```python
from build123d import *

# Parameters (mm, degrees)
BOSS_EXTRUDE1_DEPTH     = 2.54
SKETCH2_W               = 100.584
SKETCH2_H               = 101.6
BOSS_EXTRUDE2_DEPTH     = 152.4
SKETCH4_W               = 97.79508
SKETCH4_H               = 98.81108
CUT_EXTRUDE1_DEPTH      = 190.5
SKETCH6_R               = 3.175
CUT_EXTRUDE2_DEPTH      = 203.856506729
CUT_EXTRUDE4_DEPTH      = 82.182271537
CUT_EXTRUDE4_DEPTH_BACK = 183.782271537


with BuildPart() as part:
    # Sketch1 → Boss-Extrude1 (new body)
    with BuildSketch(Plane(origin=(0, 0, 0), x_dir=(1, 0, 0), z_dir=(0, 1, 0))):
        Polygon((76.035493271, -131.982271537), (152.235493271, 0), (76.035493271, 131.982271537), (-76.364506729, 131.982271537), (-152.564506729, 0), (-76.364506729, -131.982271537), align=None)
    extrude(amount=BOSS_EXTRUDE1_DEPTH)

    # Sketch2 → Boss-Extrude2 (add)
    with BuildSketch(Plane(origin=(0, 2.54, 0), x_dir=(1, 0, 0), z_dir=(0, 1, 0))):
        Rectangle(SKETCH2_W, SKETCH2_H)
    extrude(amount=BOSS_EXTRUDE2_DEPTH)

    # Sketch4 → Cut-Extrude1 (cut)
    with BuildSketch(Plane(origin=(0, 154.94, 0), x_dir=(1, 0, 0), z_dir=(0, 1, 0))):
        Rectangle(SKETCH4_W, SKETCH4_H)
    extrude(amount=-CUT_EXTRUDE1_DEPTH, mode=Mode.SUBTRACT)

    # Sketch6 → Cut-Extrude2 (cut, through all)
    with BuildSketch(Plane(origin=(50.292, 0, 0), x_dir=(0, 0, -1), z_dir=(1, 0, 0))):
        with Locations((0, 142.24)):
            Circle(SKETCH6_R)
    extrude(amount=-CUT_EXTRUDE2_DEPTH, mode=Mode.SUBTRACT)

    # Sketch7 → Cut-Extrude4 (cut, two sides)
    with BuildSketch(Plane(origin=(0, 0, -50.8), x_dir=(-1, 0, 0), z_dir=(0, 0, -1))) as cut_extrude4_sk:
        with BuildLine():
            Line((-50.292, 675.458034637), (-50.292, 154.94))
            ThreePointArc((-50.292, 154.94), (0, 104.648), (50.292, 154.94))
            Line((50.292, 154.94), (50.292, 675.458034637))
            Line((50.292, 675.458034637), (50.292, 1716.494103911))
            Line((50.292, 1716.494103911), (-50.292, 1716.494103911))
            Line((-50.292, 1716.494103911), (-50.292, 675.458034637))
        make_face()
    extrude(amount=CUT_EXTRUDE4_DEPTH, mode=Mode.SUBTRACT)
    extrude(cut_extrude4_sk.sketch, amount=-CUT_EXTRUDE4_DEPTH_BACK, mode=Mode.SUBTRACT)


solid = part.part
```
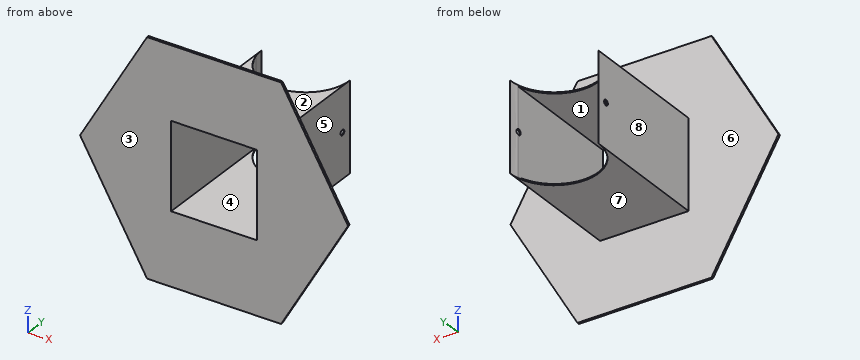
Read the model definition and answer for the solid it produces. Units are mm, in the model's axes. Face numbers are marked on the shaded views. A direction names the side the tool comes from. Give positions to 0.01 mm unless a question says otherwise; leave off trailing zeros. Loops run counter-clockwise (first coordinate to the right, second up) from the corner with the lowest first, then second, coordinate; pieces in that order, holes last.
Item 1: Find the intervals of material crossed by line 1 along X through (y, z) = (110.5, 28.5); line 2 along Z through (x, y) = (-35.5, 68); line 3 along Z through (x, y) = (-49.35, 142.24) (3 decimals), in increasing order.
Item 2: The part is cut by section A-A (y = 73.5). Write down the section's boundary in (x, z), and give its area (3 significant figures).
Item 3: The part is cut by section D-D (x = 105.5). Write down the section's boundary in (y, z), and give its area (3 significant figures).
Item 4: The mould has two halves that part along Z. Classify the marked faces 1, 2 and 3: released by +Z, released by -Z, zero draft, split by the parting line, or undercut.
Item 5: For the marked faces 4, 5, 6, 7 and 8, determine the directions among +Z, -Z, +X, -X, +Y, -Y from which every point of the face is accessible in a straight line to the end or side of a thin tool.
Item 6: The part is cut by section B-B (x = 0). Write down the section's boundary in (y, z), and give its area (3 significant figures).
Item 7: The part is cut by section C-C (z = 19.5). Write down the section's boundary in (x, y), and give its area (3 significant figures).
Item 8: Each of these flat-tipped pins is pushed along its axis until it touches: pin 1 Ø5 at (x, y) = (20, 71.5) entering from +Z; pin 2 Ø8.5 at (y, z) = (142.24, 0) entering from -X; pin 3 Ø3 at (y, z) = (29, 51.5) entering from +X; pin 4 Ø8 at (x, z) = (119.5, 68.5) entering from -Y. Where does it stop, or does it pass through?
Taken from the geometry:
1. line 1: x = -50.29 to -48.9, 48.9 to 50.29
1. line 2: z = -50.8 to -49.41, 49.41 to 50.8
1. line 3: z = -50.8 to -3.175, 3.175 to 50.8
2. outline: (-50.29, -50.8) - (50.29, -50.8) - (50.29, 50.8) - (-50.29, 50.8) - close; hole (-48.9, -49.41) - (48.9, -49.41) - (48.9, 49.41) - (-48.9, 49.41) - close
2. area: 556 mm2
3. outline: (0, -80.95) - (2.54, -80.95) - (2.54, 80.95) - (0, 80.95) - close
3. area: 411 mm2
4. face 1: undercut
4. face 2: released by +Z
4. face 3: zero draft
5. face 4: +Y, -Y
5. face 5: +Z, -Z, +X, +Y
5. face 6: +Y
5. face 7: -Z, +X, -X, +Y
5. face 8: +Z, -Z, -X, +Y
6. outline: (0, -131.98) - (2.54, -131.98) - (2.54, -50.8) - (104.65, -50.8) - (104.65, -49.41) - (0, -49.41) - close; (0, 49.41) - (104.65, 49.41) - (104.65, 50.8) - (2.54, 50.8) - (2.54, 131.98) - (0, 131.98) - close
6. area: 704 mm2
7. outline: (-141.31, 0) - (-48.9, 0) - (-48.9, 143.18) arc R50.29 cw to (-50.29, 154.94) - (-50.29, 2.54) - (-141.31, 2.54) - close; (48.9, 0) - (140.98, 0) - (140.98, 2.54) - (50.29, 2.54) - (50.29, 154.94) arc R50.29 cw to (48.9, 143.18) - close
7. area: 872 mm2
8. pin 1: stops at z = 50.8
8. pin 2: stops at x = -50.29
8. pin 3: stops at x = 50.29
8. pin 4: passes through
